The figure shows three views and two pictorial views of one solid part (mm, origin at its lowest corner). Answer the questions. Give positions to 0.01 mm unless a question says otherwise; leave off trailing zeros. Loops run counter-clockwise (first coordinate to the right, second up) from the corner with the lowest first, then second, coordinate; pieces in that order, holes last. Notation, with made-up numbers: (-38.75, 55) - (-16.75, 55) arc R18 cw to (-16.75, 77) - close; hole circle Ø3 at (11, 41). An arc over 180 degrees is marked (long way). Use a Markdown table: item, result. Add a question column.
Item 1: A cutting plane is placed at B-B (y = 58.5). Determine the outline of the cut face in (x, z), plus the area to 3 significant figures.
Item 2: Each of these flat-tipped pins is pushed along its axis until it touches: P1, Ø1.9, axis at x = 130.175, y = 12.7, coming from the -Z side; P2, Ø1.9, axis at y = 89.5, z = 3.5, coming from the -X side; P3, Ø1.9, axis at y = 92, z = 2, coming from the +X side. Where does it stop, or does it pass through?
Item 3: Consider probe 1 along X at (y, z) = (254, 4); probe 2 along Y at (x, z) = (130.5, 3.25); probe 3 along X at (y, z) = (21.5, 1.75). Determine where each line is inside the solid, lowest interval first. Write a range as [from, to].
Item 4: A cutting plane is placed at A-A (z = 1.25). Give the number of separate pieces and of enclosed holes in the cut face, plus the area to 3 significant figures.
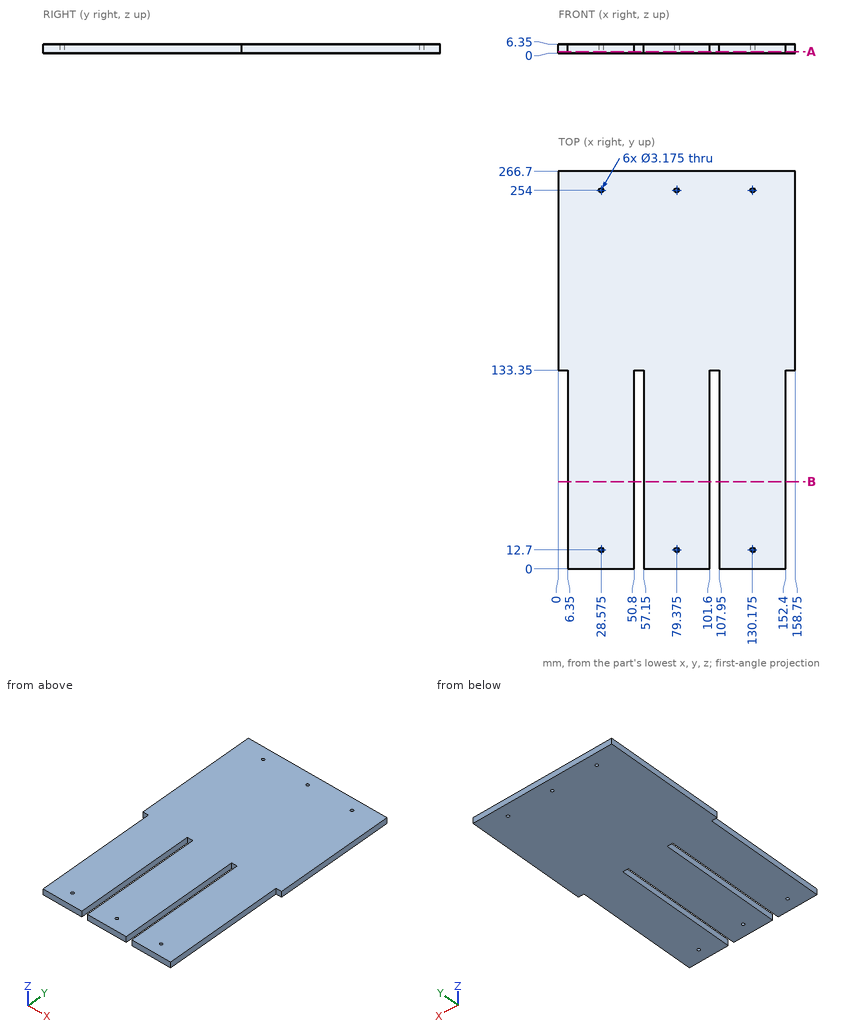
Geometry says:
| question | item | result |
|---|---|---|
| 1 | outline | (6.35, 0) - (50.8, 0) - (50.8, 6.35) - (6.35, 6.35) - close; (57.15, 0) - (101.6, 0) - (101.6, 6.35) - (57.15, 6.35) - close; (107.95, 0) - (152.4, 0) - (152.4, 6.35) - (107.95, 6.35) - close |
| 1 | area | 847 mm² |
| 2 | P1 | through |
| 2 | P2 | x = 6.35 |
| 2 | P3 | x = 152.4 |
| 3 | probe 1 | [0, 26.99], [30.16, 77.79], [80.96, 128.59], [131.76, 158.75] |
| 3 | probe 2 | [0, 11.15], [14.25, 252.45], [255.55, 266.7] |
| 3 | probe 3 | [6.35, 50.8], [57.15, 101.6], [107.95, 152.4] |
| 4 | separate pieces | 1 |
| 4 | enclosed holes | 6 |
| 4 | area | 38,900 mm² |
